```python
from build123d import *

# Parameters (mm, degrees)
SKETCH1_W           = 8
SKETCH1_H           = 80
BOSS_EXTRUDE1_DEPTH = 3
BOSS_EXTRUDE2_DEPTH = 8
FILLET1_R           = 2


with BuildPart() as part:
    # Sketch1 → Boss-Extrude1 (new body)
    with BuildSketch(Plane(origin=(0, 0, 0), x_dir=(1, 0, 0), z_dir=(0, 1, 0))):
        Rectangle(SKETCH1_W, SKETCH1_H)
    extrude(amount=BOSS_EXTRUDE1_DEPTH)

    # Sketch1<3> → Boss-Extrude2 (add)
    with BuildSketch(Plane(origin=(0, 0, 0), x_dir=(1, 0, 0), z_dir=(0, 1, 0))):
        with BuildLine():
            ThreePointArc((-70, -30), (-67.071067812, -37.071067812), (-60, -40))
            Line((-60, -40), (-4, -40))
            Line((-4, -40), (-4, 40))
            Line((-4, 40), (-60, 40))
            ThreePointArc((-60, 40), (-67.071067812, 37.071067812), (-70, 30))
            Line((-70, 30), (-70, -30))
        make_face()
        with BuildLine():
            Line((4, 40), (4, -40))
            Line((4, -40), (60, -40))
            ThreePointArc((60, -40), (67.071067812, -37.071067812), (70, -30))
            Line((70, -30), (70, 30))
            ThreePointArc((70, 30), (67.071067812, 37.071067812), (60, 40))
            Line((60, 40), (4, 40))
        make_face()
    extrude(amount=BOSS_EXTRUDE2_DEPTH)

    # Fillet1
    fillet1_edges = [part.edges().sort_by_distance(p)[0] for p in [
        (-32, 8, -40),
        (-70, 8, 0),
        (-67.071067812, 8, -37.071067812),
        (-67.071067812, 8, 37.071067812),
        (-32, 8, 40),
        (67.071067812, 8, 37.071067812),
        (67.071067812, 8, -37.071067812),
        (32, 8, -40),
        (70, 8, 0),
        (32, 8, 40),
    ]]
    fillet(fillet1_edges, radius=FILLET1_R)


solid = part.part
```
Geometry: final body of the model. Coordinates: model frame, mm. A direction names the side the tool comes from. Round coordinates to 2 decimals unless told otherwise and drop trailing zeros. Write each loop counter-clockwise with the first axis right and the second up, starting at its lowest first coordinate (ties: lowest second). Pieces come first, ordered by that corner, then holes. Notation, with made-up numbers: (84, 39.5) -> (101, 39.5) arc R23 ccw to (101, 49.5) -> close; hole circle Ø8 at (8, 16.5). An arc over 180 degrees is marked (long way). Return JSON: item names as keys, results as strings.
Q1. Section B-B on z = 1. Return the cut outline in (x, y).
From the geometry:
{"outline": "(-70, 0) -> (70, 0) -> (70, 6) arc R2 ccw to (68, 8) -> (4, 8) -> (4, 3) -> (-4, 3) -> (-4, 8) -> (-68, 8) arc R2 ccw to (-70, 6) -> close"}
Q2. First-contact query: pin 1 Ø9 at (x, z) = (1.5, -4) entering from +Y. Flat tip, straight axial feed; report the tip coordinate or a pass-through.
From the geometry:
{"pin 1": "y = 8"}
Q3. Ray query, line 1 (X direction, y = 4, z = 27.5); line 2 (X direction, y = 1.75, z = 36); line 3 (X direction, y = 7.5, z = -6.5). Return the intervals inside material, ascending.
From the geometry:
{"line 1": "-70 to -4, 4 to 70", "line 2": "-68 to 68", "line 3": "-69.32 to -4, 4 to 69.32"}
Q4. Set-up query: faces 4 (the flat face through (-4, 5, 1)), 5 (the flat face through (-1, 0, -1)). Return all of +Z, -Z, +X, -X, +Y, -Y with unobstructed straight access to the full face (end or side cutting, diameter ignored); none if empty.
From the geometry:
{"face 4": "+Z, -Z, +Y", "face 5": "+Z, -Z, +X, -X, -Y"}
Q5. Mould query, pull axis X, two halves, no side actions, for faces 1 (the flat face through (0, 3, -1)), 2 (the flat face through (-36, 8, -1)), 3 (the cylindrical face through (67.15, 2.96, -36.99)). Classes: +X half, -X half, draft (parallel to the pull), parting line (faces both ways), or undercut.
From the geometry:
{"face 1": "undercut", "face 2": "draft", "face 3": "+X half"}
Q6. Section A-A on y = 4.75. Return the cut outline in (x, z), and give its area (3 significant figures).
From the geometry:
{"outline": "(-70, -30) arc R10 ccw to (-60, -40) -> (-4, -40) -> (-4, 40) -> (-60, 40) arc R10 ccw to (-70, 30) -> close; (4, -40) -> (60, -40) arc R10 ccw to (70, -30) -> (70, 30) arc R10 ccw to (60, 40) -> (4, 40) -> close", "area": "10,500 mm2"}
